Verification items for the finished model (mm, model axes). A direction names the side the tool comes from. Give positions to 0.01 mm unless a question says otherwise; leave off trailing zeros. Order: outer loops, then holes, each group sorted by start corner. A loop starts at its lowest first (then second) coordinate and runs counter-clockwise, first axis right, second up.
from build123d import *
from build123d.topology import SkipClean

# Parameters (mm, degrees)
SKETCH_1_W               = 100
SKETCH_1_H               = 15
EXTRUDE_1_DEPTH          = 50
SKETCH_2_R               = 1.1
CUT_EXTRUDE_1_DEPTH      = 72.107313267
SKETCH_3_W               = 12
SKETCH_3_H               = 30
CUT_EXTRUDE_5_DEPTH      = 15
CUT_EXTRUDE_5_DEPTH_BACK = 15
EXTRUDE_2_DEPTH          = 4.5
CUT_EXTRUDE_START        = -2.5
SKETCH_5_R               = 2.7
CUT_EXTRUDE_2_DEPTH      = 12.5
SKETCH_6_R               = 1.4
CUT_EXTRUDE_4_DEPTH      = 67.304223093
MIRROR_2_DEPTH           = 8
MIRROR_START             = 5.5
MIRROR_2_2_DEPTH         = 4.5
MIRROR_START_2           = 8
MIRROR_2_3_DEPTH         = 2
MIRROR_4_DEPTH           = 8
MIRROR_START_3           = 42
MIRROR_4_2_DEPTH         = 8
MIRROR_4_3_DEPTH         = 34
MIRROR_4_4_DEPTH         = 4.5
MIRROR_START_4           = 40
MIRROR_4_5_DEPTH         = 4.5
MIRROR_4_6_DEPTH         = 2
MIRROR_4_7_DEPTH         = 2


# Read off the part's stored shape, not the designer's step: the mirror step, the mirror step
with BuildPart() as part:
    # Sketch 1 → Extrude 1 (new body)
    with BuildSketch(Plane(origin=(0, 0, 0), x_dir=(1, 0, 0), z_dir=(0, 1, 0))):
        Rectangle(SKETCH_1_W, SKETCH_1_H)
    extrude(amount=EXTRUDE_1_DEPTH)

    # Sketch 2 → Cut-Extrude 1 (cut, through all)
    with BuildSketch(Plane(origin=(0, 50, 0), x_dir=(1, 0, 0), z_dir=(0, 1, 0))):
        with Locations(Location((-45, -2.5, 0), (0, 0, 270))):
            Circle(SKETCH_2_R)
        with Locations(Location((45, -2.5, 0), (0, 0, 90))):
            Circle(SKETCH_2_R)
    extrude(amount=-CUT_EXTRUDE_1_DEPTH, mode=Mode.SUBTRACT)

    # Sketch 3 → Cut-Revolve 1 (revolve, cut)
    with BuildSketch(Plane.XY.offset(7.5)):
        with Locations((-44, 25)):
            Rectangle(SKETCH_3_W, SKETCH_3_H)
    cut_revolve_1 = revolve(axis=Axis((-50, 10, 7.5), (0, 1, 0)), mode=Mode.SUBTRACT)

    # Mirror 1: Cut-Revolve 1 across plane
    add(cut_revolve_1.mirror(Plane.ZY), mode=Mode.SUBTRACT)

    # Sketch 10 → Cut-Extrude 5 (cut, two sides: drawn at the far end of the back side and taken through both)
    with BuildSketch(Plane.XZ.offset(-25).offset(-CUT_EXTRUDE_5_DEPTH_BACK)):
        with BuildLine():
            Line((-5, 2.5), (5, 2.5))
            ThreePointArc((5, 2.5), (8.535533906, 3.964466094), (10, 7.5))
            Line((10, 7.5), (-10, 7.5))
            ThreePointArc((-10, 7.5), (-8.535533906, 3.964466094), (-5, 2.5))
        make_face()
    extrude(amount=CUT_EXTRUDE_5_DEPTH + CUT_EXTRUDE_5_DEPTH_BACK, mode=Mode.SUBTRACT)

    # Sketch 7 → Extrude 2 (add)
    with BuildSketch(Plane(origin=(0, 40, 0), x_dir=(1, 0, 0), z_dir=(0, 1, 0))):
        with BuildLine():
            Line((-9, -7.5), (-1, -7.5))
            ThreePointArc((-1, -7.5), (-5, -11.5), (-9, -7.5))
        make_face()
    extrude(amount=EXTRUDE_2_DEPTH)

    # Sketch 5 → Cut-Extrude 2 (cut)
    with BuildSketch(Plane(origin=(0, 44.5, 0), x_dir=(1, 0, 0), z_dir=(0, 1, 0)).offset(CUT_EXTRUDE_START)):
        with Locations((-5, -7.5)):
            Circle(SKETCH_5_R)
    extrude(amount=CUT_EXTRUDE_2_DEPTH, mode=Mode.SUBTRACT)

    # Sketch 6 → Cut-Extrude 4 (cut, through all)
    with BuildSketch(Plane(origin=(0, 42, 0), x_dir=(1, 0, 0), z_dir=(0, 1, 0))):
        with Locations(Location((-5, -7.5, 0), (0, 0, 270))):
            Circle(SKETCH_6_R)
    extrude(amount=-CUT_EXTRUDE_4_DEPTH, mode=Mode.SUBTRACT)

    # Mirror 2 outline → Mirror 2 (cut)
    with BuildSketch(Plane(origin=(0, 0, 0), x_dir=(1, 0, 0), z_dir=(0, 1, 0))):
        with BuildLine():
            ThreePointArc((-6.4, -7.5), (-5, -6.1), (-3.6, -7.5))
            Line((-3.6, -7.5), (-2.3, -7.5))
            ThreePointArc((-2.3, -7.5), (-5, -4.8), (-7.7, -7.5))
            Line((-7.7, -7.5), (-6.4, -7.5))
        make_face()
    extrude(amount=MIRROR_2_DEPTH, mode=Mode.SUBTRACT)

    # Mirror 2 2 outline → Mirror 2 2 (add)
    with BuildSketch(Plane(origin=(0, 0, 0), x_dir=(1, 0, 0), z_dir=(0, 1, 0)).offset(MIRROR_START)):
        with BuildLine():
            Line((-1, -7.5), (-2.3, -7.5))
            ThreePointArc((-2.3, -7.5), (-5, -10.2), (-7.7, -7.5))
            Line((-7.7, -7.5), (-9, -7.5))
            ThreePointArc((-9, -7.5), (-5, -11.5), (-1, -7.5))
        make_face()
    extrude(amount=MIRROR_2_2_DEPTH)

    # Mirror 2 3 outline → Mirror 2 3 (add)
    with BuildSketch(Plane(origin=(0, 0, 0), x_dir=(1, 0, 0), z_dir=(0, 1, 0)).offset(MIRROR_START_2)):
        with BuildLine():
            Line((-2.3, -7.5), (-3.6, -7.5))
            ThreePointArc((-3.6, -7.5), (-5, -8.9), (-6.4, -7.5))
            Line((-6.4, -7.5), (-7.7, -7.5))
            ThreePointArc((-7.7, -7.5), (-5, -10.2), (-2.3, -7.5))
        make_face()
    extrude(amount=MIRROR_2_3_DEPTH)

    # Mirror 4 outline → Mirror 4 (cut)
    with BuildSketch(Plane(origin=(0, 0, 0), x_dir=(1, 0, 0), z_dir=(0, 1, 0))):
        with BuildLine():
            ThreePointArc((7.7, -7.5), (5, -4.8), (2.3, -7.5))
            Line((2.3, -7.5), (7.7, -7.5))
        make_face()
    extrude(amount=MIRROR_4_DEPTH, mode=Mode.SUBTRACT)

    # Mirror 4 2 outline → Mirror 4 2 (cut)
    with BuildSketch(Plane(origin=(0, 0, 0), x_dir=(1, 0, 0), z_dir=(0, 1, 0)).offset(MIRROR_START_3)):
        with BuildLine():
            ThreePointArc((7.7, -7.5), (5, -4.8), (2.3, -7.5))
            Line((2.3, -7.5), (7.7, -7.5))
        make_face()
    extrude(amount=MIRROR_4_2_DEPTH, mode=Mode.SUBTRACT)

    # Mirror 4 3 outline → Mirror 4 3 (cut)
    with BuildSketch(Plane(origin=(0, 0, 0), x_dir=(1, 0, 0), z_dir=(0, 1, 0)).offset(MIRROR_START_2)):
        with BuildLine():
            Line((3.6, -7.5), (6.4, -7.5))
            ThreePointArc((6.4, -7.5), (5, -6.1), (3.6, -7.5))
        make_face()
    extrude(amount=MIRROR_4_3_DEPTH, mode=Mode.SUBTRACT)

    # Mirror 4 4 outline → Mirror 4 4 (add)
    with BuildSketch(Plane(origin=(0, 0, 0), x_dir=(1, 0, 0), z_dir=(0, 1, 0)).offset(MIRROR_START)):
        with BuildLine():
            Line((9, -7.5), (7.7, -7.5))
            ThreePointArc((7.7, -7.5), (5, -10.2), (2.3, -7.5))
            Line((2.3, -7.5), (1, -7.5))
            ThreePointArc((1, -7.5), (5, -11.5), (9, -7.5))
        make_face()
    extrude(amount=MIRROR_4_4_DEPTH)

    # Mirror 4 5 outline → Mirror 4 5 (add)
    with SkipClean():  # the faces are left unmerged after this step: merging them gives an invalid solid
        with BuildSketch(Plane(origin=(0, 0, 0), x_dir=(1, 0, 0), z_dir=(0, 1, 0)).offset(MIRROR_START_4)):
            with BuildLine():
                Line((9, -7.5), (7.7, -7.5))
                ThreePointArc((7.7, -7.5), (5, -10.2), (2.3, -7.5))
                Line((2.3, -7.5), (1, -7.5))
                ThreePointArc((1, -7.5), (5, -11.5), (9, -7.5))
            make_face()
        extrude(amount=MIRROR_4_5_DEPTH)

    # Mirror 4 6 outline → Mirror 4 6 (add)
    with SkipClean():  # the faces are left unmerged after this step: merging them gives an invalid solid
        with BuildSketch(Plane(origin=(0, 0, 0), x_dir=(1, 0, 0), z_dir=(0, 1, 0)).offset(MIRROR_START_2)):
            with BuildLine():
                Line((7.7, -7.5), (6.4, -7.5))
                ThreePointArc((6.4, -7.5), (5, -8.9), (3.6, -7.5))
                Line((3.6, -7.5), (2.3, -7.5))
                ThreePointArc((2.3, -7.5), (5, -10.2), (7.7, -7.5))
            make_face()
        extrude(amount=MIRROR_4_6_DEPTH)

    # Mirror 4 7 outline → Mirror 4 7 (add)
    with SkipClean():  # the faces are left unmerged after this step: merging them gives an invalid solid
        with BuildSketch(Plane(origin=(0, 0, 0), x_dir=(1, 0, 0), z_dir=(0, 1, 0)).offset(MIRROR_START_4)):
            with BuildLine():
                Line((7.7, -7.5), (6.4, -7.5))
                ThreePointArc((6.4, -7.5), (5, -8.9), (3.6, -7.5))
                Line((3.6, -7.5), (2.3, -7.5))
                ThreePointArc((2.3, -7.5), (5, -10.2), (7.7, -7.5))
            make_face()
        extrude(amount=MIRROR_4_7_DEPTH)


solid = part.part
(1) Section check D-D, the plane x = 12. Enter the section's corners in (y, z).
Solved:
outline: (0, -7.5) - (50, -7.5) - (50, 7.5) - (0, 7.5) - close
(2) Go/stop test with flat-tipped pins: pin 1 (1.3 mm diameter, centred on x = -45, z = 2.5, fed in from -Y); pin 2 (2 mm diameter, centred on x = 11.5, y = 35, fed in from +Z); pin 3 (4.5 mm diameter, centred on x = -5.5, z = 8.5, fed in from -Y); pin 4 (5 mm diameter, centred on x = 5, z = 7.5, fed in from +Y). Record where each tip stops, or that it passes through.
Solved:
pin 1: passes through
pin 2: stops at z = 7.5
pin 3: stops at y = 5.5
pin 4: stops at y = 42
(3) Section check A-A, the plane y = 34. Enter the section's corners in (x, z).
Solved:
outline: (-50, -7.5) - (50, -7.5) - (50, -4.5) arc R12 cw to (38, 7.5) - (10, 7.5) arc R5 cw to (5, 2.5) - (-5, 2.5) arc R5 cw to (-10, 7.5) - (-38, 7.5) arc R12 cw to (-50, -4.5) - close
(4) Scan lines: line 1 (X direction, y = 5, z = 2.5); line 2 (Y direction, x = 3, z = 2.75); line 3 (Z direction, x = 45, y = 42). Record each from-to range of solid material in increasing order.
Solved:
line 1: x = -50 to -46.1, -43.9 to 43.9, 46.1 to 50
line 2: y = 0 to 10, 40 to 50
line 3: z = -7.5 to 1.4, 3.6 to 7.5
(5) Release check for a two-part mould opening along Y. For faces 1 (the flat face through (45, 10, 1)), 2 (the flat face through (-50, 25, -5)), 3 (the flat face through (-1, 0, 0)), 4 (the flat face through (-45, 40, 1)) record: pulls with the +Y half, pulls with the -Y half, needs draft (parallel to the pull), parting line crosses it, or undercut.
Solved:
face 1: undercut
face 2: needs draft
face 3: pulls with the -Y half
face 4: undercut
(6) Section check C-C, the plane z = -2. Enter the section's corners in (x, y), then the cut area to 3 significant figures.
Solved:
outline: (-50, 0) - (50, 0) - (50, 10) - (42.67, 10) - (42.67, 40) - (50, 40) - (50, 50) - (-50, 50) - (-50, 40) - (-42.67, 40) - (-42.67, 10) - (-50, 10) - close
area: 4,560 mm2
(7) Section check B-B, the plane x = 45. Enter the section's corners in (y, z).
Solved:
outline: (0, -7.5) - (50, -7.5) - (50, 1.4) - (40, 1.4) - (40, -3.41) - (10, -3.41) - (10, 1.4) - (0, 1.4) - close; (0, 3.6) - (10, 3.6) - (10, 7.5) - (0, 7.5) - close; (40, 3.6) - (50, 3.6) - (50, 7.5) - (40, 7.5) - close
(8) Set-up check for faces 5 (the flat face through (-4, 8, 9)), 6 (the cylindrical face through (-41.42, 25.21, -0.89)), 7 (the cylindrical face through (8.5, 25.21, 3.93)): record each of +Z, -Z, +X, -X, +Y, -Y from which the full face is reachable in a straight line by a thin tool's end or side.
Solved:
face 5: -Y
face 6: +Z, -X
face 7: +Z
